Could you check a few things on this model? Use its own coordinates, in mm. Face numbers are marked on the shaded views. Coordinates: 2 decimals unless noted, no trailing zeros. Write each loop counter-clockwise with the first axis right and the second up, starting at its lowest first coordinate (ties: lowest second). Pieces come first, ordered by that corner, then holes.
```python
from build123d import *

# Parameters (mm, degrees)
ESQUISSE1_R        = 1.5
ESQUISSE1_R_2      = 2
BOSS_EXTRU_1_DEPTH = 3


with BuildPart() as part:
    # Esquisse1 → Boss.-Extru.1 (new body)
    with BuildSketch(Plane.XY):
        with BuildLine():
            Line((-47, 50), (73, 50))
            ThreePointArc((73, 50), (80.071067812, 47.071067812), (83, 40))
            Line((83, 40), (83, 10))
            ThreePointArc((83, 10), (80.071067812, 2.928932188), (73, 0))
            Line((73, 0), (47, 0))
            Line((47, 0), (34.119561541, 0))
            ThreePointArc((34.119561541, 0), (33.41245476, 0.292893219), (33.119561541, 1))
            Line((33.119561541, 1), (33.119561541, 9.539430389))
            ThreePointArc((33.119561541, 9.539430389), (33.326632605, 10.148744513), (33.862088945, 10.505715989))
            ThreePointArc((33.862088945, 10.505715989), (30, 40), (26.137911055, 10.505715989))
            ThreePointArc((26.137911055, 10.505715989), (26.673367395, 10.148744513), (26.880438459, 9.539430389))
            Line((26.880438459, 9.539430389), (26.880438459, 1))
            ThreePointArc((26.880438459, 1), (26.58754524, 0.292893219), (25.880438459, 0))
            Line((25.880438459, 0), (-25.880438459, 0))
            ThreePointArc((-25.880438459, 0), (-26.58754524, 0.292893219), (-26.880438459, 1))
            Line((-26.880438459, 1), (-26.880438459, 9.539430389))
            ThreePointArc((-26.880438459, 9.539430389), (-26.673367395, 10.148744513), (-26.137911055, 10.505715989))
            ThreePointArc((-26.137911055, 10.505715989), (-30, 40), (-33.862088945, 10.505715989))
            ThreePointArc((-33.862088945, 10.505715989), (-33.326632605, 10.148744513), (-33.119561541, 9.539430389))
            Line((-33.119561541, 9.539430389), (-33.119561541, 1))
            ThreePointArc((-33.119561541, 1), (-33.41245476, 0.292893219), (-34.119561541, 0))
            Line((-34.119561541, 0), (-47, 0))
            ThreePointArc((-47, 0), (-49.871560265, 0.42116178), (-52.501242243, 1.649171671))
            ThreePointArc((-52.501242243, 1.649171671), (-52.723609687, 2.016078741), (-52.579733522, 2.420266478))
            Line((-52.579733522, 2.420266478), (-49.464466094, 5.535533906))
            ThreePointArc((-49.464466094, 5.535533906), (-49.464466094, 8.363961031), (-52.292893219, 8.363961031))
            Line((-52.292893219, 8.363961031), (-55.181690934, 5.475163315))
            ThreePointArc((-55.181690934, 5.475163315), (-55.617572947, 5.335541283), (-55.98446771, 5.60917548))
            ThreePointArc((-55.98446771, 5.60917548), (-56.742809582, 7.746633308), (-57, 10))
            Line((-57, 10), (-57, 40))
            ThreePointArc((-57, 40), (-54.071067812, 47.071067812), (-47, 50))
        make_face()
        with Locations((-6, 25)):
            Circle(ESQUISSE1_R, mode=Mode.SUBTRACT)
        with Locations((-54, 25)):
            Circle(ESQUISSE1_R, mode=Mode.SUBTRACT)
        with Locations((6, 25)):
            Circle(ESQUISSE1_R, mode=Mode.SUBTRACT)
        with Locations((50, 39)):
            Circle(ESQUISSE1_R_2, mode=Mode.SUBTRACT)
        with Locations((10, 39)):
            Circle(ESQUISSE1_R_2, mode=Mode.SUBTRACT)
        with Locations((-10, 39)):
            Circle(ESQUISSE1_R_2, mode=Mode.SUBTRACT)
        with Locations((-50, 39)):
            Circle(ESQUISSE1_R_2, mode=Mode.SUBTRACT)
        with BuildLine():
            Line((76.105551896, 31.349468926), (77.188840425, 31.158455931))
            ThreePointArc((77.188840425, 31.158455931), (77.834344291, 30.747224614), (78, 30))
            Line((78, 30), (74.527036447, 10.30384494))
            ThreePointArc((74.527036447, 10.30384494), (74.11580513, 9.658341073), (73.368580516, 9.492685364))
            Line((73.368580516, 9.492685364), (72.285291988, 9.68369836))
            ThreePointArc((72.285291988, 9.68369836), (71.639788121, 10.094929677), (71.474132412, 10.842154291))
            Line((71.474132412, 10.842154291), (74.947095966, 30.538309351))
            ThreePointArc((74.947095966, 30.538309351), (75.358327282, 31.183813217), (76.105551896, 31.349468926))
        make_face(mode=Mode.SUBTRACT)
    extrude(amount=BOSS_EXTRU_1_DEPTH)


solid = part.part
```
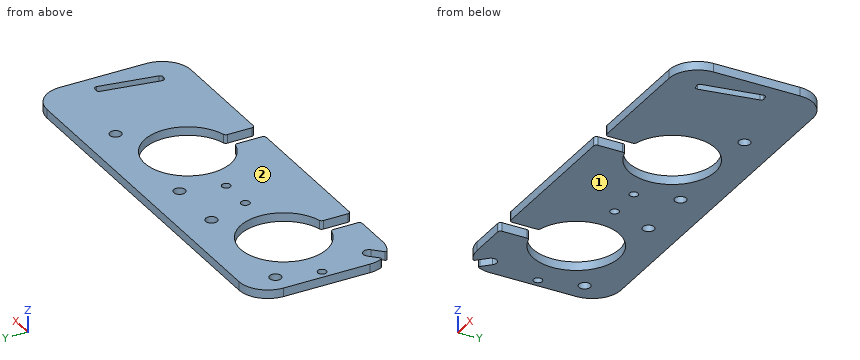
Item 1: I want a section at D-D, the plane x = 6. List the corners of the cut face in (y, z) for me.
Item 2: I want a section at A-A, the plane y = 25. List the corners of the cut face in (x, z) for me.
Item 3: Will these pins go through, and if not, where does the flat tip stop? pin 1 Ø12 at (x, y) = (56, 42) entering from -Z; pin 2 Ø1.5 at (y, z) = (4, 1.5) entering from -X.
Item 4: I want a section at B-B, the plane x = -37.5. List the corners of the cut face in (y, z) for me.
Item 5: If I drill on line 1 along X through (y, z) = (5, 2.45); line 2 along Y through (x, z) = (6, 1.5); line 3 along Y through (x, z) = (-50, 1.7), over which ranges is the centre line in solid material (lowest first)?
Item 6: I want a section at C-C, the plane y = 19.5. List the corners of the cut face in (x, z) for me, then the cut area to 3 significant figures.
Item 7: If we mould it in two halves opening along Z, with no side actions, what happens to the marked faces 1 and 2? For each: released by +Z, released by -Z, zero draft, split by the parting line, or undercut.
Taken from the geometry:
1. outline: (0, 0) - (23.5, 0) - (23.5, 3) - (0, 3) - close; (26.5, 0) - (50, 0) - (50, 3) - (26.5, 3) - close
2. outline: (-57, 0) - (-55.5, 0) - (-55.5, 3) - (-57, 3) - close; (-52.5, 0) - (-45, 0) - (-45, 3) - (-52.5, 3) - close; (-15, 0) - (-7.5, 0) - (-7.5, 3) - (-15, 3) - close; (-4.5, 0) - (4.5, 0) - (4.5, 3) - (-4.5, 3) - close; (7.5, 0) - (15, 0) - (15, 3) - (7.5, 3) - close; (45, 0) - (73.97, 0) - (73.97, 3) - (45, 3) - close; (77.12, 0) - (83, 0) - (83, 3) - (77.12, 3) - close
3. pin 1: stops at z = 0
3. pin 2: stops at x = -51.75
4. outline: (0, 0) - (12.01, 0) - (12.01, 3) - (0, 3) - close; (37.99, 0) - (50, 0) - (50, 3) - (37.99, 3) - close
5. line 1: x = -50 to -33.12, -26.88 to 26.88, 33.12 to 81.66
5. line 2: y = 0 to 23.5, 26.5 to 50
5. line 3: y = 0.46 to 5, 8.75 to 37, 41 to 49.54
6. outline: (-57, 0) - (-43.96, 0) - (-43.96, 3) - (-57, 3) - close; (-16.04, 0) - (16.04, 0) - (16.04, 3) - (-16.04, 3) - close; (43.96, 0) - (73, 0) - (73, 3) - (43.96, 3) - close; (76.15, 0) - (83, 0) - (83, 3) - (76.15, 3) - close
6. area: 243 mm2
7. face 1: released by -Z
7. face 2: released by +Z
